Geometry: final body of the model. Coordinates: model frame, mm. Face numbers are marked on the shaded views. A direction names the side the tool comes from. Coordinates: 2 decimals unless noted, no trailing zeros. Order: outer loops, then holes, each group sorted by start corner. A loop starts at its lowest first (then second) coordinate and runs counter-clockwise, first axis right, second up. Notation, with made-up numbers: M 25,-30 L 33,-30 A22 ccw 33,0 Z; hole C 64.5,89.5 d4. An arc over 180 degrees is marked long. Write item = value, one per line. Start each with the question number.
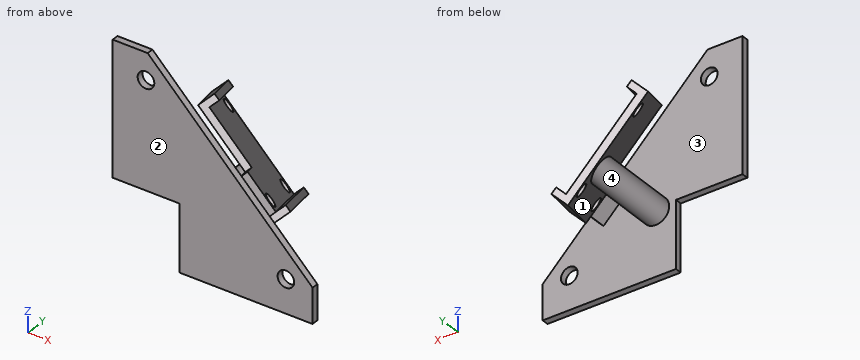
```python
from build123d import *

# Parameters (mm, degrees)
SKETCH_1_R                  = 2.5
EXTRUDE_1_DEPTH             = 2
SKETCH_2_R                  = 2
EXTRUDE_3_DEPTH             = 2
EXTRUDE_4_REACH             = 93.431
SKETCH_4_R                  = 4
EXTRUDE_5_REACH             = 93.431
EXTRUDE_6_REACH             = 56.956
EXTRUDE_6_DIRECTION_2_DEPTH = 3
SKETCH_7_R                  = 2.5
EXTRUDE_8_DEPTH             = 3
CUT_EXTRUDE_1_DEPTH         = 3


with BuildPart() as part:
    # Sketch 1 → Extrude 1 (new body)
    with BuildSketch(Plane(origin=(0, 0, 0), x_dir=(1, 0, 0), z_dir=(0, 1, 0))):
        Polygon((10.502525317, -60), (60, -10.502525317), (60, 0), (20, 0), (20, -20), (0, -20), (0, -60), align=None)
        with Locations(Location((10, -52, 0), (0, 0, 270))):
            Circle(SKETCH_1_R, mode=Mode.SUBTRACT)
        with Locations(Location((52, -10, 0), (0, 0, 270))):
            Circle(SKETCH_1_R, mode=Mode.SUBTRACT)
    extrude(amount=EXTRUDE_1_DEPTH)



with BuildPart() as body_2:
    # Sketch 2 → Extrude 3 (new body)
    with BuildSketch(Plane(origin=(24.318415307, 24.081140456, 24.318415307), x_dir=(-0.7071067811865475, 0, 0.7071067811865476), z_dir=(0.5792279653395701, 0.5735764363510444, 0.57922796533957))):
        Polygon((-3, 16.786030205), (-15, 16.786030205), (-15, -13.213969795), (15, -13.213969795), (15, 9.786030205), (-3, 9.786030205), align=None)
        with Locations(Location((-12, -10.213969795, 0), (0, 0, 180))):
            Circle(SKETCH_2_R, mode=Mode.SUBTRACT)
        with Locations(Location((12, -10.213969795, 0), (0, 0, 180))):
            Circle(SKETCH_2_R, mode=Mode.SUBTRACT)
        with Locations(Location((-12, 13.786030205, 0), (0, 0, 180))):
            Circle(SKETCH_2_R, mode=Mode.SUBTRACT)
    extrude(amount=EXTRUDE_3_DEPTH)


with BuildPart() as part_1:
    add(part.part)

    add(body_2.part)  # Extrude 4 merges body 2
    # Extrude 4: up to this plane
    extrude_4_end = Plane(origin=(24.318415307, 24.081140456, 24.318415307), z_dir=(0.5792279653395702, 0.5735764363510445, 0.5792279653395699))
    # Sketch 4 → Extrude 4 (add, up to the surface)
    with BuildSketch(Plane(origin=(0, 2, 0), x_dir=(1, 0, 0), z_dir=(0, 1, 0)), mode=Mode.PRIVATE) as extrude_4_sk1:
        with Locations(Location((26.030164055, -18.959096243, 0), (0, 0, 315))):
            Circle(SKETCH_4_R)
    extrude_4_tool1 = split(extrude(extrude_4_sk1.sketch, amount=EXTRUDE_4_REACH, mode=Mode.PRIVATE), bisect_by=extrude_4_end, keep=Keep.BOTH, mode=Mode.PRIVATE)
    add(extrude_4_tool1.solids().sort_by_distance((26.030164, 2, 18.959096))[0])

    # Sketch 5 → Extrude 5 (add, up to next)
    with BuildSketch(Plane(origin=(0, 2, 0), x_dir=(1, 0, 0), z_dir=(0, 1, 0)), mode=Mode.PRIVATE) as extrude_5_sk1:
        Polygon((41.733091591, -20.519888156), (33.247810217, -29.00516953), (34.406266148, -30.16362546), (42.891547522, -21.678344086), align=None)
    extrude_5_tool1 = extrude(extrude_5_sk1.sketch, amount=EXTRUDE_5_REACH, mode=Mode.PRIVATE) - part_1.part
    add(extrude_5_tool1.solids().sort_by_distance((38.069679, 2, 25.341757))[0])

    # Extrude 6: up to this face of the body (flat: up to its plane)
    extrude_6_end = Plane(part_1.part.faces().sort_by_distance((24.757422588, 23.562214363, 24.393270957))[0])
    # Sketch 6 → Extrude 6 (add, up to the picked face)
    with BuildSketch(Plane(origin=(25.476871238, 25.228293329, 25.476871238), x_dir=(0.45107473692648714, 0.36633593098762024, -0.8138363271408656), z_dir=(0.5792279653395703, 0.5735764363510442, 0.5792279653395701)), mode=Mode.PRIVATE) as extrude_6_sk1:
        Polygon((-7.506940922, 18.527137818), (-17.792853619, -2.044687575), (-19.581708001, -1.150260384), (-9.295795304, 19.421565009), align=None)
    extrude_6_tool1 = split(extrude(extrude_6_sk1.sketch, amount=-EXTRUDE_6_REACH, mode=Mode.PRIVATE), bisect_by=extrude_6_end, keep=Keep.BOTH, mode=Mode.PRIVATE)
    # Sketch 6 → Extrude 6 (add, up to the picked face)
    with BuildSketch(Plane(origin=(25.476871238, 25.228293329, 25.476871238), x_dir=(0.45107473692648714, 0.36633593098762024, -0.8138363271408656), z_dir=(0.5792279653395703, 0.5735764363510442, 0.5792279653395701)), mode=Mode.PRIVATE) as extrude_6_sk2:
        Polygon((19.325874808, 5.110729953), (5.909466943, -21.722085777), (7.698321325, -22.616512968), (21.11472919, 4.216302762), align=None)
    extrude_6_tool2 = split(extrude(extrude_6_sk2.sketch, amount=-EXTRUDE_6_REACH, mode=Mode.PRIVATE), bisect_by=extrude_6_end, keep=Keep.BOTH, mode=Mode.PRIVATE)
    add(extrude_6_tool1.solids().sort_by(Axis((13.468011, 26.632295, 36.095428), (-0.5792279653395703, -0.5735764363510442, -0.5792279653395701)))[0])
    add(extrude_6_tool2.solids().sort_by(Axis((37.514957, 23.765263, 14.88754), (-0.5792279653395703, -0.5735764363510442, -0.5792279653395701)))[0])

    # Sketch 6 → Extrude 6 direction 2 (add)
    with BuildSketch(Plane(origin=(25.476871238, 25.228293329, 25.476871238), x_dir=(0.45107473692648714, 0.36633593098762024, -0.8138363271408656), z_dir=(0.5792279653395703, 0.5735764363510442, 0.5792279653395701))):
        Polygon((-7.506940922, 18.527137818), (-17.792853619, -2.044687575), (-19.581708001, -1.150260384), (-9.295795304, 19.421565009), align=None)
        Polygon((19.325874808, 5.110729953), (5.909466943, -21.722085777), (7.698321325, -22.616512968), (21.11472919, 4.216302762), align=None)
    extrude(amount=EXTRUDE_6_DIRECTION_2_DEPTH)

    # Sketch 7 → Extrude 8 (add)
    with BuildSketch(Plane(origin=(0, 2, 0), x_dir=(1, 0, 0), z_dir=(0, 1, 0))):
        Polygon((60, 0), (20, 0), (20, -20), (0, -20), (0, -60), (10.502525317, -60), (60, -10.502525317), align=None)
        with Locations(Location((10, -52, 0), (0, 0, 270))):
            Circle(SKETCH_7_R, mode=Mode.SUBTRACT)
        with Locations(Location((52, -10, 0), (0, 0, 270))):
            Circle(SKETCH_7_R, mode=Mode.SUBTRACT)
    extrude(amount=EXTRUDE_8_DEPTH)

    # Sketch 10 → Cut-Extrude 1 (cut)
    with BuildSketch(Plane.XZ):
        Polygon((20, 0), (60, 0), (60, 10.502525317), (10.502525317, 60), (0, 60), (0, 20), (20, 20), align=None)
    extrude(amount=-CUT_EXTRUDE_1_DEPTH, mode=Mode.SUBTRACT)


solid = part_1.part
```
Item 1: Section query B-B on x = 52. Output: boundary loops of the cut face in (y, z), and give its area (3 significant figures).
Item 2: Section query D-D on z = 37.5. Output: boundary loops of the cut face in (x, y), and give its area (3 significant figures).
Item 3: First-contact query: pin 1 (4 mm diameter, centred on x = 40, y = 31, fed in from -Z); pin 2 (2 mm diameter, centred on x = 8.5, y = 4.5, fed in from -Z); pin 3 (2 mm diameter, centred on x = 20.5, y = 21, fed in from +Z); pin 4 (5 mm diameter, centred on x = 36.5, z = 6.5, fed in from +Y). Flat tips, straight axial feed; report the tip coordinate or a pass-through.
Item 4: Reachability of the marked faces 1 and 2 from +Z, -Z, +X, -X, +Y, -Y: full face, straight path, thin tool, end or side. Return the list, or none.
Item 5: Section query A-A on z = 52. Output: boundary loops of the cut face in (x, y).
Item 6: Section query C-C on y = 7.5. Output: boundary loops of the cut face in (x, z).
Item 7: Material intervals for probe 1 along X at (y, z) = (4.5, 10); probe 2 along Y at (x, z) = (10.5, 24), sorted ascending. Write a range as [from, to].
Item 8: Draft query along Z for the marked faces 3 and 4. Return one class per face: pulls with the +Z half, pulls with the -Z half, needs draft (parallel to the pull), parting line crosses it, or undercut.
Ans:
q1.outline = M 3,0 L 5,0 L 5,7.5 L 3,7.5 Z; M 3,12.5 L 5,12.5 L 5,18.5 L 3,18.5 Z
q1.area = 27.0 mm^2
q2.outline = M 0,3 L 33,3 L 33,5 L 0,5 Z; M 13.46,21.74 L 19.07,16.06 L 21.39,17.21 L 16.29,22.37 L 16.29,27.6 L 13.46,30.45 Z
q2.area = 104 mm^2
q3.pin_1 = through
q3.pin_2 = 20
q3.pin_3 = 41.23
q3.pin_4 = 5
q4.face_1 = none
q4.face_2 = +Z, -Z, +X, -X, -Y
q5.outline = M 0,3 L 7.5,3 L 7.5,5 L 0,5 Z; M 12.5,3 L 18.5,3 L 18.5,5 L 12.5,5 Z
q6.outline = C 26.03,18.96 d8; M 33.25,29.01 L 41.73,20.52 L 42.89,21.68 L 34.41,30.16 Z
q7.probe_1 = [20, 49.5], [54.5, 60]
q7.probe_2 = [3, 5]
q8.face_3 = needs draft
q8.face_4 = undercut
